Could you check a few things on this model? Use its own coordinates, in mm. Face numbers are marked on the shaded views. A direction names the side the tool comes from. Give positions to 0.01 mm unless a question says otherwise; leave off trailing zeros. Order: outer loops, then holes, each group sorted by start corner. A loop starts at its lowest first (then second) coordinate and runs counter-clockwise, first axis right, second up.
(1) If I drill on probe 1 along Y at (x, z) = (10, -1); probe 2 along X at (y, z) = (69.5, 40); probe 3 along Y at (x, z) = (10, 2), over which ranges is the centre line in solid material (lowest first)?
(2) Will these pins go through, and if not, where does the flat tip stop? pin 1 (2 mm diameter, centred on x = 21.5, y = 103.5, fed in from +Z); pin 2 (4 mm diameter, centred on x = 53, y = 48.5, fed in from -Z); pin 3 (2 mm diameter, centred on x = 149.5, y = 96.5, fed in from +Z).
(3) If we mould it in two halves opening along Y, with no side actions, what happens to the marked faces 1, 2 and 3? For each: released by +Y, released by -Y, zero draft, split by the parting line, or undercut.
(4) Imagine slicing it at A-A, the plane x = 115.5. Write out the boundary of the cut face in (y, z).
(5) On a 3-axis mill with a long thin cutter (end or side, diameter ignored), from which of +Z, -Z, +X, -X, +Y, -Y can I reach the whole of each face in a straight line? I mean the marked faces 4 and 5. Say none if no direction works.
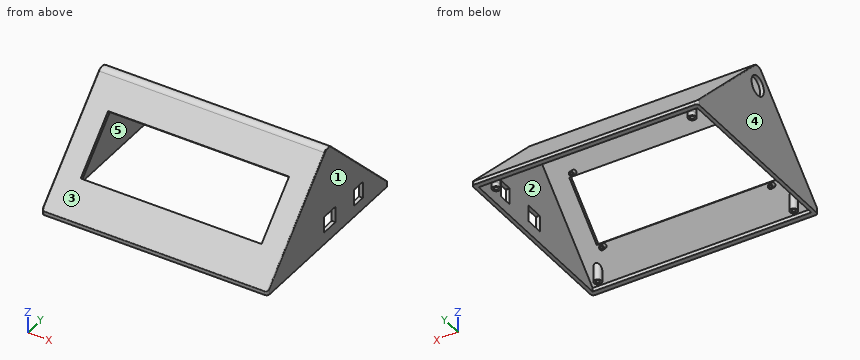
from build123d import *

# Parameters (mm, degrees)
F1_DEPTH  = 150
F2_T      = -2.5
F4_W      = 120
F4_H      = 41
F5_DEPTH  = 3
F6_R      = 5
F8_R      = 1.5
F8_R_2    = 0.75
F9_DEPTH  = 6.5
F10_R     = 2.5
F10_R_2   = 1.5
F12_R     = 2.5
F12_R_2   = 1.25
F13_REACH = 68.6406103068
F14_W     = 150
F14_H     = 127.2792206136
F14_W_2   = 145
F14_H_2   = 120.2081528017
F15_DEPTH = 2.5
F16_R     = 2.5
F16_R_2   = 1.25
F18_R     = 2
F19_R     = 0.5
F7_W      = 9
F7_H      = 11
F7_W_2    = 12.1
F7_H_2    = 10.7
F20_DEPTH = 3
F21_R     = 0.5
F22_R     = 0.5
F23_R     = 6.5
F24_DEPTH = 2.5
F25_R     = 2.5
F25_R_2   = 1.25
F26_DEPTH = 2.5


with BuildPart() as f1:
    # F0 (on Right) → F1 (new body)
    with BuildSketch(Plane.YZ):
        Polygon((63.6396103068, 63.6396103068), (0, 0), (127.2792206136, 0), align=None)
    extrude(amount=F1_DEPTH)

    # F2
    f2_openings = [f1.faces().sort_by_distance(p)[0] for p in [
        (75, 63.63961, 0),
    ]]
    offset(amount=F2_T, openings=f2_openings, kind=Kind.INTERSECTION)

    # F4 (on offset) → F5 (cut)
    with BuildSketch(Plane(origin=(0, 0, 0), x_dir=(1, 0, 0), z_dir=(0, -0.7071067812, 0.7071067812))):
        with Locations((75, 45)):
            Rectangle(F4_W, F4_H)
    extrude(amount=-F5_DEPTH, mode=Mode.SUBTRACT)

    # F6
    f6_edges = [f1.edges().sort_by_distance(p)[0] for p in [
        (75, 63.63961, 63.63961),
    ]]
    fillet(f6_edges, radius=F6_R)

    # F8 (on face) → F9 (join)
    with BuildSketch(Plane(origin=(0, 0, 0), x_dir=(1, 0, 0), z_dir=(0, -0.7071067812, 0.7071067812))):
        with Locations((131, 67.5)):
            Circle(F8_R)
        with Locations((131, 67.5)):
            Circle(F8_R_2, mode=Mode.SUBTRACT)
        with Locations((131, 22.5)):
            Circle(F8_R)
        with Locations((131, 22.5)):
            Circle(F8_R_2, mode=Mode.SUBTRACT)
        with Locations((19, 67.5)):
            Circle(F8_R)
        with Locations((19, 67.5)):
            Circle(F8_R_2, mode=Mode.SUBTRACT)
        with Locations((19, 22.5)):
            Circle(F8_R)
        with Locations((19, 22.5)):
            Circle(F8_R_2, mode=Mode.SUBTRACT)
    extrude(amount=-F9_DEPTH)

    # F10 (on face) → F11 (join, up to the last surface of F1)
    with BuildSketch(Plane(origin=(0, 0, 0), x_dir=(1, 0, 0), z_dir=(0, 0, -1))):
        with Locations((10, -10)):
            Circle(F10_R)
        with Locations((10, -10)):
            Circle(F10_R_2, mode=Mode.SUBTRACT)
    extrude(until=Until.LAST, dir=(0, 0, 1))

    f13_end = Plane(origin=(75.2456023398, 33.6766976894, 30.1411637835), x_dir=(0, 0.7071067812, 0.7071067812), z_dir=(0, 0.7071067812, -0.7071067812))
    # F12 (on face) → F13 (join, up to a plane its end follows)
    with BuildSketch(Plane(origin=(0, 0, 0), x_dir=(1, 0, 0), z_dir=(0, 0, -1))):
        with Locations((10, -10)):
            Circle(F12_R)
        with Locations((10, -10)):
            Circle(F12_R_2, mode=Mode.SUBTRACT)
        with Locations((140, -10)):
            Circle(F12_R)
        with Locations((140, -10)):
            Circle(F12_R_2, mode=Mode.SUBTRACT)
    f13_long = extrude(amount=-F13_REACH, mode=Mode.PRIVATE)
    add(split(f13_long, bisect_by=f13_end, keep=Keep.TOP, mode=Mode.PRIVATE))

    # F14 (on face) → F15 (join)
    with BuildSketch(Plane(origin=(0, 0, 0), x_dir=(1, 0, 0), z_dir=(0, 0, -1))):
        with Locations((75, -63.6396103068)):
            Rectangle(F14_W, F14_H)
        with Locations((75, -63.6396103068)):
            Rectangle(F14_W_2, F14_H_2, mode=Mode.SUBTRACT)
    extrude(amount=F15_DEPTH)

    # F16 (on Top) → F17 (join, up to the next surface of F1)
    with BuildSketch(Plane.XY):
        with Locations((140, 117.279)):
            Circle(F16_R)
        with Locations((140, 117.279)):
            Circle(F16_R_2, mode=Mode.SUBTRACT)
        with Locations((10, 117.279)):
            Circle(F16_R)
        with Locations((10, 117.279)):
            Circle(F16_R_2, mode=Mode.SUBTRACT)
    extrude(until=Until.NEXT)

    # F18
    f18_edges = [f1.edges().sort_by_distance(p)[0] for p in [
        (150, 127.279221, -1.25),
        (150, 0, -1.25),
        (0, 0, -1.25),
        (0, 127.279221, -1.25),
    ]]
    fillet(f18_edges, radius=F18_R)

    # F19
    f19_edges = [f1.edges().sort_by_distance(p)[0] for p in [
        (0, 31.052038, 31.052038),
    ]]
    fillet(f19_edges, radius=F19_R)

    # F7 (on face) → F20 (cut)
    with BuildSketch(Plane.YZ.offset(150)):
        with Locations((95.7792206136, 10.65)):
            Rectangle(F7_W, F7_H)
        with Locations((65.4042206136, 10.95)):
            Rectangle(F7_W_2, F7_H_2)
    extrude(amount=-F20_DEPTH, mode=Mode.SUBTRACT)

    # F21
    f21_edges = [f1.edges().sort_by_distance(p)[0] for p in [
        (148.75, 91.279221, 16.15),
        (148.75, 100.279221, 16.15),
    ]]
    fillet(f21_edges, radius=F21_R)

    # F22
    f22_edges = [f1.edges().sort_by_distance(p)[0] for p in [
        (148.75, 59.354221, 16.3),
        (148.75, 71.454221, 16.3),
    ]]
    fillet(f22_edges, radius=F22_R)

    # F23 (on face) → F24 (cut)
    with BuildSketch(Plane(origin=(0, 0, 0), x_dir=(0, -1, 0), z_dir=(-1, 0, 0))):
        with Locations((-64, 47.5)):
            Circle(F23_R)
    extrude(amount=-F24_DEPTH, mode=Mode.SUBTRACT)

    # F25 (on face) → F26 (join)
    with BuildSketch(Plane(origin=(0, 0, 0), x_dir=(1, 0, 0), z_dir=(0, 0, -1))):
        with Locations((10, -10)):
            Circle(F25_R)
        with Locations((10, -10)):
            Circle(F25_R_2, mode=Mode.SUBTRACT)
        with Locations((140, -10)):
            Circle(F25_R)
        with Locations((140, -10)):
            Circle(F25_R_2, mode=Mode.SUBTRACT)
        with Locations((10, -117.279)):
            Circle(F25_R)
        with Locations((10, -117.279)):
            Circle(F25_R_2, mode=Mode.SUBTRACT)
        with Locations((140, -117.279)):
            Circle(F25_R)
        with Locations((140, -117.279)):
            Circle(F25_R_2, mode=Mode.SUBTRACT)
    extrude(amount=F26_DEPTH)


solid = f1.part
Answer block:
1. probe 1: y = 0 to 3.54, 7.5 to 8.75, 11.25 to 12.5, 114.78 to 116.03, 118.53 to 119.78, 123.74 to 127.28
1. probe 2: x = 0 to 2.5, 147.5 to 150
1. probe 3: y = 2 to 5.54, 7.5 to 8.75, 11.25 to 12.5, 114.78 to 116.03, 118.53 to 119.78, 121.74 to 125.28
2. pin 1: stops at z = 24.78
2. pin 2: stops at z = 44.55
2. pin 3: stops at z = 31.78
3. face 1: zero draft
3. face 2: undercut
3. face 3: released by -Y
4. outline: (0, -2.5) - (3.54, -2.5) - (3.54, 0) - (19.09, 15.56) - (17.32, 17.32) - (0.15, 0.15) arc R0.5 ccw to (0, -0.21) - close; (46.32, 46.32) - (48.08, 44.55) - (63.64, 60.1) - (123.74, 0) - (123.74, -2.5) - (127.28, -2.5) - (127.28, -0.21) arc R0.5 ccw to (127.13, 0.15) - (67.18, 60.1) arc R5 ccw to (60.1, 60.1) - close
5. face 4: +Z, -Z, -X, +Y, -Y
5. face 5: -Z
